Autodesk Inventor part; units mm, degrees
ref_plane "YZ Plane" through (0, 0, 0) normal (1, 0, 0) x (0, 1, 0)
ref_plane "XZ Plane" through (0, 0, 0) normal (0, 1, 0) x (-1, 0, 0)
ref_plane "XY Plane" through (0, 0, 0) normal (0, 0, 1) x (1, 0, 0)
sketch "Sketch1" plane through (0, 0, 0) normal (0, 0, 1) x (1, 0, 0)
  circle A0 centre (0, 0) radius 15 construction
  circle A1 centre (0, 0) radius 26 construction
  line L0 (3.5, 37) -> (-3.5, 37) construction
  line L1 (-3.5, 37) -> (-3.5, 15) construction
  line L2 (-3.5, 15) -> (3.5, 15) construction
  line L3 (3.5, 15) -> (3.5, 37) construction
  line L4 (3.5, 37) -> (-3.5, 15) construction
  line L5 (-3.5, 37) -> (3.5, 15) construction
  line L6 (-6.5, 16) -> (-6.5, 40) construction
  line L7 (-6.5, 40) -> (6.5, 40) construction
  line L8 (6.5, 40) -> (6.5, 16) construction
  circle A2 centre (0, 0) radius 17.2699 construction
  line L9 (-16.5, 16) -> (-16.5, 50) construction
  line L10 (-16.5, 50) -> (16.5, 50) construction
  line L11 (16.5, 50) -> (16.5, 16) construction
  circle A3 centre (0, 0) radius 23 construction
  line L12 (-25, 26) -> (25, 26) construction
  line L13 (-25, 30) -> (25, 30) construction
  line L14 (-25, 22) -> (25, 22) construction
  line L15 (-35.0513, -39.2894) -> (-51.5513, -10.7106) construction
  line L16 (-31.391, -25.6292) -> (-37.891, -14.3708) construction
  line L17 (-5.6064, -22.2894) -> (-35.0513, -39.2894) construction
  line L18 (-51.5513, -10.7106) -> (-22.1064, 6.2894) construction
  line L19 (-37.891, -14.3708) -> (-17.1064, -2.3708) construction
  line L20 (-10.6064, -13.6292) -> (-31.391, -25.6292) construction
  line L21 (-30.2929, -21.5311) -> (-11.2404, -10.5311) construction
  line L22 (-11.2404, -10.5311) -> (-14.7404, -4.4689) construction
  line L23 (-14.7404, -4.4689) -> (-33.7929, -15.4689) construction
  line L24 (-33.7929, -15.4689) -> (-11.2404, -10.5311) construction
  line L25 (-30.2929, -21.5311) -> (-14.7404, -4.4689) construction
  line L26 (-33.7929, -15.4689) -> (-30.2929, -21.5311) construction
  line L27 (-13.4808, -36.6506) -> (-38.4808, 6.6506) construction
  line L28 (-10.0167, -34.6506) -> (-35.0167, 8.6506) construction
  line L29 (-6.5526, -32.6506) -> (-31.5526, 10.6506) construction
  line L30 (51.5513, -10.7106) -> (35.0513, -39.2894) construction
  line L31 (37.891, -14.3708) -> (31.391, -25.6292) construction
  line L32 (22.1064, 6.2894) -> (51.5513, -10.7106) construction
  line L33 (35.0513, -39.2894) -> (5.6064, -22.2894) construction
  line L34 (31.391, -25.6292) -> (10.6064, -13.6292) construction
  line L35 (17.1064, -2.3708) -> (37.891, -14.3708) construction
  line L36 (33.7929, -15.4689) -> (14.7404, -4.4689) construction
  line L37 (14.7404, -4.4689) -> (11.2404, -10.5311) construction
  line L38 (11.2404, -10.5311) -> (30.2929, -21.5311) construction
  line L39 (30.2929, -21.5311) -> (14.7404, -4.4689) construction
  line L40 (33.7929, -15.4689) -> (11.2404, -10.5311) construction
  line L41 (30.2929, -21.5311) -> (33.7929, -15.4689) construction
  line L42 (38.4808, 6.6506) -> (13.4808, -36.6506) construction
  line L43 (35.0167, 8.6506) -> (10.0167, -34.6506) construction
  line L44 (31.5526, 10.6506) -> (6.5526, -32.6506) construction
  line L45 (-16.5, 16.0234) -> (-16.5, 50)
  line L46 (-16.5, 50) -> (16.5, 50)
  line L47 (16.5, 50) -> (16.5, 16.0234)
  line L48 (-6.5, 16) -> (-6.5, 40)
  line L49 (-6.5, 40) -> (6.5, 40)
  line L50 (6.5, 40) -> (6.5, 16)
  line L51 (-22.1267, 6.2777) -> (-51.5513, -10.7106)
  line L52 (-51.5513, -10.7106) -> (-46.5513, -19.3708)
  line L53 (-46.5513, -19.3708) -> (-17.1064, -2.3708)
  line L54 (46.5513, -19.3708) -> (51.5513, -10.7106)
  line L55 (51.5513, -10.7106) -> (22.1267, 6.2777)
  line L56 (17.1064, -2.3708) -> (46.5513, -19.3708)
  line L57 (37.891, -14.3708) -> (31.391, -25.6292)
  arc A4 (-6.5, 16) -> (-17.1064, -2.3708) centre (0, 0) ccw
  arc A5 (-16.5, 16.0234) -> (-22.1267, 6.2777) centre (0, 0) ccw
  arc A6 (17.1064, -2.3708) -> (6.5, 16) centre (0, 0) ccw
  arc A7 (22.1267, 6.2777) -> (16.5, 16.0234) centre (0, 0) ccw
  point P0 (0, 26)
  point P1 (0, 26)
  point P2 (0, 26)
  point P3 (0, 30)
  point P4 (0, 22)
  point P5 (-25.9808, -15)
  point P6 (-22.5167, -13)
  point P7 (-22.5167, -13)
  point P8 (-22.5167, -13)
  point P9 (-5.6267, -22.3011)
  point P10 (-19.0526, -11)
  point P11 (25.9808, -15)
  point P12 (22.5167, -13)
  point P13 (22.5167, -13)
  point P14 (22.5167, -13)
  point P15 (19.0526, -11)
  dimension "d1" = 52
  dimension "d0" = 30
  dimension "d2" = 7
  dimension "d4" = 3
  dimension "d5" = 3
  dimension "d6" = 3
  dimension "d7" = 16
  dimension "d8" = 10
  dimension "d9" = 10
  dimension "d11" = 10
  dimension "d12" = 3
  dimension "d13" = 50
  dimension "d14" = 4
  dimension "d15" = 4
  dimension "d16" = 50
  dimension "d17" = 50
  dimension "d20" = 360
extrude "Extrusion3" add sketch "Sketch1" along normal blind 70
sketch "Sketch6" plane through (16.5, 16.0234, 0) normal (1, 0, 0) x (0, 0, -1)
  line L0 (0, 9.9766) -> (-71.7893, 9.9766) construction
  line L1 (-70, 0) -> (-70, 33.9766) construction
  point P0 (0, -16.0234)
  point P1 (0, 9.9766)
  point P2 (-58, 9.9766)
  point P3 (-12, 9.9766)
  dimension "d46" = 12
  dimension "d47" = 12
sketch "Sketch7" plane through (0, 0, 70) normal (0, 0, 1) x (1, 0, 0)
  line L0 (-22.1267, 6.2777) -> (-51.5513, -10.7106)
  line L1 (-51.5513, -10.7106) -> (-51.5513, 50)
  line L2 (-51.5513, 50) -> (-16.5, 50)
  line L3 (16.5, 16.0234) -> (16.5, 50)
  line L4 (16.5, 50) -> (51.5513, 50)
  line L5 (51.5513, 50) -> (51.5513, -10.7106)
  arc A0 (-16.5, 16.0234) -> (-22.1267, 6.2777) centre (0, 0) ccw
  line L6 (-16.5, 50) -> (-16.5, 16.0234)
  arc A1 (22.1267, 6.2777) -> (16.5, 16.0234) centre (0, 0) ccw
  line L7 (51.5513, -10.7106) -> (22.1267, 6.2777)
  line L8 (51.5513, 50) -> (51.5513, -10.7106)
  point P0 (0, 0)
  point P1 (16.5, 26)
extrude "Extrusion5" add sketch "Sketch7" against normal blind 24
hole "Hole3" at (16.5, 26, 58) at (16.5, 26, 12) direction (-1, 0, 0) diameter 8.2 end through all
hole "Hole4" at (-51.5513, 26, 58) direction (1, 0, 0) diameter 8.2 end through all
sketch "Sketch10" plane through (-22.1267, 6.2777, 46) normal (-0.5, 0.866, 0) x (0.866, 0.5, 0)
  line L0 (-9.9766, 46) -> (-9.9766, -2.7834) construction
  line L1 (-33.9766, 0) -> (0, 0) construction
  line L2 (-33.9766, 46) -> (-33.9766, -24) construction
  line L3 (-33.9766, 11) -> (0, 11) construction
  line L4 (0, 46) -> (0, 0) construction
  point P0 (16.0234, 46)
  point P1 (-9.9766, 46)
  point P2 (-9.9766, 11)
hole "Hole5" at (-30.7667, 1.2894, 35) direction (0.5, -0.866, 0) diameter 8.2 end through all
sketch "Sketch11" plane through (51.5513, -10.7106, 46) normal (0.5, 0.866, 0) x (0.866, -0.5, 0)
  line L0 (-24, 46) -> (-24, 0) construction
  line L1 (-33.9766, 0) -> (0, 0) construction
  line L2 (0, 46) -> (0, -24) construction
  line L3 (0, 11) -> (-34, 11) construction
  line L4 (-34, 46) -> (-34, -24) construction
  point P0 (-50, 46)
  point P1 (-24, 11)
hole "Hole6" at (30.7667, 1.2894, 35) direction (-0.5, -0.866, 0) diameter 8.2 end through all
fillet "Fillet2" radius 2 10 edges at (-36.839, -2.2164, 46) (-19.9186, 11.5, 46) (-16.5, 33.0117, 46) (-16.5, 16.0234, 23) (-22.1267, 6.2777, 23) (16.5, 16.0234, 23) (22.1267, 6.2777, 23) (16.5, 33.0117, 46) (19.9186, 11.5, 46) (36.839, -2.2164, 46)
fillet "Fillet3" radius 10 1 edges at (0, 50, 0)
chamfer "Chamfer1" distance 20 angle 45 2 edges at (49.0513, -15.0407, 0) (-49.0513, -15.0407, 0)
sketch "Sketch12" plane through (-51.5513, 50, 70) normal (0, 1, 0) x (1, 0, 0)
  line L0 (0, 0) -> (0, 24) construction
  line L1 (0, 12) -> (103.1025, 12) construction
  line L2 (103.1025, 0) -> (103.1025, 24) construction
  line L3 (0, 24) -> (33.0513, 24) construction
  line L4 (16.5256, 24) -> (16.5256, 0) construction
  line L5 (5, 0) -> (34.4449, 0) construction
  line L6 (70.0513, 24) -> (103.1025, 24) construction
  line L7 (86.5769, 24) -> (86.5769, 0) construction
  line L8 (103.1025, 0) -> (0, 0) construction
  point P0 (51.5513, 70)
  point P1 (86.5769, 12)
  point P2 (16.5256, 12)
hole "Hole7" at (35.0256, 50, 58) at (-35.0256, 50, 58) direction (0, -1, 0) diameter 8.2 end through all
sketch "Sketch13" plane through (0, 0, 70) normal (0, 0, 1) x (1, 0, 0)
  line L0 (51.5513, 50) -> (-51.5513, 50) construction
  line L1 (-43.5513, 50) -> (-43.5513, -5) construction
  line L2 (0, 50) -> (0, -7.7688) construction
  point P0 (0, 0)
  point P1 (-43.5513, 42)
  point P2 (-43.5513, 15)
  point P3 (-43.5513, 42)
  point P4 (-43.5513, 15)
  point P5 (43.5513, 42)
  point P6 (43.5513, 15)
  point P7 (43.5513, 42)
  point P8 (43.5513, 15)
  dimension "d95" = 8
  dimension "d96" = 8
  dimension "d97" = 35
hole "Hole8" at (-43.5513, 42, 70) at (-43.5513, 15, 70) at (43.5513, 42, 70) at (43.5513, 15, 70) direction (0, 0, -1) diameter 8.2 end through all
sketch "Sketch14" plane through (0, 0, 70) normal (0, 0, 1) x (1, 0, 0)
  point P0 (0, 0)
sketch "Sketch15" plane through (0, 0, 70) normal (0, 0, 1) x (1, 0, 0)
  line L0 (-51.5513, 50) -> (-51.5513, -10.7106)
  line L1 (51.5513, -10.7106) -> (51.5513, 50)
  line L2 (-51.5513, -0.3388) -> (51.5513, -0.3388)
  line L3 (51.5513, -0.3388) -> (51.5513, -25.3388)
  line L4 (51.5513, -25.3388) -> (-51.5513, -25.3388)
  line L5 (-51.5513, -25.3388) -> (-51.5513, -0.3388)
  point P0 (0, 0)
  dimension "d105" = 25
extrude "Extrusion6" cut sketch "Sketch15" against normal blind 22
equation "\"d5\" = d4"
equation "\"d6\" = d4"
equation "\"d9\" = d8"
equation "\"d15\" = d14"
equation "\"d16\" = d13"
equation "\"d17\" = d16"
equation "\"d50\" = 2 * d47"
properties part number "Linear_pipe" material "ABS Plastic"
Build history of the part. All positions in model axes, mm. A direction names the side the tool comes from. Coordinates: 2 decimals unless noted, no trailing zeros. Order: outer loops, then holes, each group sorted by start corner. A loop starts at its lowest first (then second) coordinate and runs counter-clockwise, first axis right, second up. Notation, with made-up numbers: (-8, 10) - (18, 10) arc R25 cw to (18, 37) - close; hole circle Ø10 at (66.5, -31.75). An arc over 180 degrees is marked (long way). Write item = value, one per line. Start each with the question number.
1) Saw through at C-C on z = 33.5. Write the cut outline in (x, y), then the cut area to 3 significant figures.
2) Saw through at D-D on y = -13.5. Write the cut outline in (x, z).
3) Flat gauge pins, fed straight in: pin 1 Ø7.5 at (x, y) = (-43.55, 42) entering from -Z; pin 2 Ø10 at (x, y) = (-35.5, 21) entering from -Z; pin 3 Ø1 at (x, z) = (32, 35) entering from +Y; pin 4 Ø14.5 at (x, z) = (-1.5, 49) entering from -Y. Where does each tip first touch, or does it go through?
4) Two-plate mould, pull along Z, no slides. Class faces 1 (the face through (45.009, 23.505, 54.746)), 2 (the face through (0.23, 46.99, 2.85)), 3 (the face through (31.62, -10.75, 23.66)): pulls with the +Z half, pulls with the -Z half, needs draft (parallel to the pull), parting line crosses it, or undercut.
5) Saw through at A-A on y = 42. Write the cut outline in (x, z).
6) Saw through at B-B on x = 11. Write the cut outline in (y, z), then the cut area to 3 significant figures.
7) Wall check: line 1 along X through (y, z) = (19, 20.5); line 2 along Y through (x, z) = (27, 58); line 3 along Y through (x, z) = (-0.5, 54). Give the ranges that are in metal, low to high. Write a range as from..to.
8) 3-axis set-ups, long thin cutter, end or side, ignore diameter. For faces 4 (the face through (16.5, 34, 22)), 5 (the face through (14.876, 8.773, 34.51)), 6 (the face through (-49.086, -14.98, 33.804)), 7 (the face through (-19.953, 11.44, 21.692)), 8 (the face through (38, -8, 48)): which of +Z, -Z, +X, -X, +Y, -Y reach the whole face in a straight line?
From the geometry:
q1.outline = (-51.55, -10.71) - (-46.55, -19.37) - (-29.07, -9.28) - (-34.07, -0.62) - close; (-27.46, 3.2) - (-22.46, -5.46) - (-17.11, -2.37) arc R17.27 cw to (-6.5, 16) - (-6.5, 40) - (6.5, 40) - (6.5, 16) arc R17.27 cw to (17.11, -2.37) - (22.46, -5.46) - (27.46, 3.2) - (22.81, 5.88) arc R2 cw to (21.91, 7) arc R23 ccw to (17.02, 15.47) arc R2 cw to (16.5, 16.82) - (16.5, 50) - (-16.5, 50) - (-16.5, 16.82) arc R2 cw to (-17.02, 15.47) arc R23 ccw to (-21.91, 7) arc R2 cw to (-22.81, 5.88) - close; (29.07, -9.28) - (46.55, -19.37) - (51.55, -10.71) - (34.07, -0.62) - close
q1.area = 1,520 mm^2
q2.outline = (-49.94, 20) - (-36.38, 8.26) - (-36.38, 48) - (-49.94, 48) - close; (36.38, 8.26) - (49.94, 20) - (49.94, 48) - (36.38, 48) - close
q3.pin_1 = through
q3.pin_2 = 46
q3.pin_3 = -3.91
q3.pin_4 = 14.89
q4.face_1 = undercut
q4.face_2 = pulls with the -Z half
q4.face_3 = needs draft
q5.outline = (-51.55, 46) - (-47.65, 46) - (-47.65, 70) - (-51.55, 70) - close; (-39.45, 46) - (-18.5, 46) arc R2 cw to (-16.5, 44) - (-16.5, 0.2) - (16.5, 0.2) - (16.5, 44) arc R2 cw to (18.5, 46) - (39.45, 46) - (39.45, 70) - (-39.45, 70) - close; (47.65, 46) - (51.55, 46) - (51.55, 70) - (47.65, 70) - close; hole circle Ø8.2 at (-35.03, 58); hole circle Ø8.2 at (35.03, 58)
q6.outline = (13.31, 0) - (40, 0) arc R10 ccw to (50, 10) - (50, 70) - (13.31, 70) - close; hole circle Ø8.2 at (26, 12); hole circle Ø8.2 at (26, 58)
q6.area = 2,440 mm^2
q7.line_1 = -16.5..-6.5, 6.5..16.5
q7.line_2 = -0.34..21.9, 30.1..50
q7.line_3 = 40..50
q8.face_4 = -Z, +X, +Y
q8.face_5 = +Z, -Z
q8.face_6 = +Z, -Z, -X, -Y
q8.face_7 = -Z, -X, +Y
q8.face_8 = +Z, +X, -X, -Y
